Geometry check sheet. Reference: the model listing, model coordinates, mm. A direction names the side the tool comes from. Round coordinates to 2 decimals unless told otherwise and drop trailing zeros. Order: outer loops, then holes, each group sorted by start corner. A loop starts at its lowest first (then second) coordinate and runs counter-clockwise, first axis right, second up. Notation, with made-up numbers: (68, 62) -> (101, 62) arc R16 ccw to (101, 91) -> close; hole circle Ø7 at (11, 4). An arc over 180 degrees is marked (long way). Answer as a JSON object with one key per item and string values. Group by question number.
Autodesk Inventor part; units mm, degrees
ref_plane "YZ Plane" through (0, 0, 0) normal (1, 0, 0) x (0, 1, 0)
ref_plane "XZ Plane" through (0, 0, 0) normal (0, 1, 0) x (-1, 0, 0)
ref_plane "XY Plane" through (0, 0, 0) normal (0, 0, 1) x (1, 0, 0)
sketch "Sketch1" plane through (0, 0, 0) normal (0, 0, 1) x (1, 0, 0)
  line L0 (-6.5, -6.5) -> (6.5, -6.5)
  line L1 (6.5, -6.5) -> (6.5, 6.5)
  line L2 (6.5, 6.5) -> (-6.5, 6.5)
  line L3 (-6.5, 6.5) -> (-6.5, -6.5)
  line L4 (-6.5, -6.5) -> (6.5, 6.5) construction
  line L5 (6.5, -6.5) -> (-6.5, 6.5) construction
  line L6 (-5.5, 5.5) -> (5.5, 5.5)
  line L7 (5.5, 5.5) -> (5.5, -5.5)
  line L8 (5.5, -5.5) -> (-5.5, -5.5)
  line L9 (-5.5, -5.5) -> (-5.5, 5.5)
  point P0 (0, 0)
  dimension "d0" = 13
  dimension "d1" = 13
  dimension "d2" = 1
extrude "Extrusion1" add sketch "Sketch1" along normal blind 2 contours L3 L2 L1 L0 | L6 L7 L8 L9
extrude "Extrusion2" cut sketch "Sketch1" along normal blind 1 contours L6 L7 L8 L9
sketch "Sketch2" plane through (0, 0, 2) normal (0, 0, 1) x (1, 0, 0)
  line L0 (-6.5, -6.5) -> (6.5, -6.5)
  line L1 (-1, -6.5) -> (1, -6.5)
  line L2 (1, -6.5) -> (1, -2)
  line L3 (1, -2) -> (-1, -2)
  line L4 (-1, -2) -> (-1, -6.5)
  point P0 (0, 0)
  point P1 (0, -6.5)
  dimension "d7" = 2
  dimension "d8" = 4.5
  dimension "d9" = 1
extrude "Extrusion3" add sketch "Sketch2" against normal blind 5.5
sketch "Sketch3" plane through (0, 0, 0) normal (0, 0, -1) x (-1, 0, 0)
  line L0 (-5.5, 5.5) -> (5.5, 5.5)
  line L1 (-6.5, 6.5) -> (6.5, 6.5)
  line L2 (-5.5, 5.5) -> (5.5, 5.5)
  line L3 (5.5, 5.5) -> (5.5, 6.5)
  line L4 (5.5, 6.5) -> (-5.5, 6.5)
  line L5 (-5.5, 6.5) -> (-5.5, 5.5)
  point P0 (0, 0)
  dimension "d12" = 11
extrude "Extrusion4" cut sketch "Sketch3" against normal blind 1
properties part number "NV_module_lid_2" material "PET Plastic"
Item 1: Sectioned sample at D-D, the plane y = -2.5. Enter the section's corners in (x, z), then the cut area to 3 significant figures.
Item 2: Depth check by flat-ended pin: pin 1 Ø0.8 at (x, z) = (3, 0.5) entering from +Y; pin 2 Ø1.6 at (x, y) = (-2.5, 0) entering from -Z; pin 3 Ø1.6 at (x, z) = (0, -1.5) entering from +Y. Enter the tip coordinate at first touch or a pass-through.
Item 3: Mould release check, pull along X, two halves, no side actions. Record for faces 1 (the flat face through (0, 0, 2)), 2 (the flat face through (6.5, 0, 1)), 3 (the flat face through (-6.5, 0, 1)), 4 (the flat face through (3.3, -5.5, 0.5)): pulls with the +X half, pulls with the -X half, needs draft (parallel to the pull), parting line crosses it, or undercut.
Item 4: Sectioned sample at B-B, the plane y = 4. Enter the section's corners in (x, z).
Item 5: Sectioned sample at A-A, the plane z = 0.35. Enter the section's corners in (x, y), then the cut area to 3 significant figures.
Item 6: Thickness scan on L1, parallel to X at y = -3.75, z = 0.1; L2, parallel to X at y = 0, z = 0.2; L3, parallel to X at y = -5, z = -1.9. Record the ranges inside material, lowest first.
Item 7: Sectioned sample at C-C, the plane x = 2.25. Enter the section's corners in (y, z), then the cut area to 3 significant figures.
Item 8: Set-up check for faces 5 (the flat face through (-6, -1, 0)), 6 (the flat face through (6, -1, 0)), 7 (the flat face through (0, -4, -3.5)), 8 (the flat face through (-3.2, -5.5, 0.5)): record each of +Z, -Z, +X, -X, +Y, -Y from which the full face is reachable in a straight line by a thin tool's end or side.
Result:
{
 "1": {"outline": "(-6.5, 0) -> (-5.5, 0) -> (-5.5, 1) -> (-1, 1) -> (-1, -3.5) -> (1, -3.5) -> (1, 1) -> (5.5, 1) -> (5.5, 0) -> (6.5, 0) -> (6.5, 2) -> (-6.5, 2) -> close", "area": "24.0 mm2"},
 "2": {"pin 1": "stops at y = -5.5", "pin 2": "stops at z = 1", "pin 3": "stops at y = -2"},
 "3": {"face 1": "needs draft", "face 2": "pulls with the +X half", "face 3": "pulls with the -X half", "face 4": "undercut"},
 "4": {"outline": "(-6.5, 0) -> (-5.5, 0) -> (-5.5, 1) -> (5.5, 1) -> (5.5, 0) -> (6.5, 0) -> (6.5, 2) -> (-6.5, 2) -> close"},
 "5": {"outline": "(-6.5, -6.5) -> (6.5, -6.5) -> (6.5, 6.5) -> (5.5, 6.5) -> (5.5, -5.5) -> (1, -5.5) -> (1, -2) -> (-1, -2) -> (-1, -5.5) -> (-5.5, -5.5) -> (-5.5, 6.5) -> (-6.5, 6.5) -> close", "area": "44.0 mm2"},
 "6": {"L1": "x = -6.5 to -5.5, -1 to 1, 5.5 to 6.5", "L2": "x = -6.5 to -5.5, 5.5 to 6.5", "L3": "x = -1 to 1"},
 "7": {"outline": "(-6.5, 0) -> (-5.5, 0) -> (-5.5, 1) -> (6.5, 1) -> (6.5, 2) -> (-6.5, 2) -> close", "area": "14.0 mm2"},
 "8": {"face 5": "-Z, -X, +Y, -Y", "face 6": "-Z, +X, +Y, -Y", "face 7": "-Z, +X, -X, +Y, -Y", "face 8": "-Z, +Y"}
}
